Check sheet for the drawn part. Datum: minimum x, y, z corner. Units: mm. A direction names the side the tool comes from. Round coordinates to 2 decimals unless told otherwise and drop trailing zeros. Order: outer loops, then holes, each group sorted by start corner. A loop starts at its lowest first (then second) coordinate and runs counter-clockwise, first axis right, second up. Notation, with made-up numbers: (74.5, -36) -> (122.5, -36) arc R20 ccw to (122.5, -26) -> close; hole circle Ø3 at (81, 21). An arc over 180 degrees is marked (long way). Answer in a Markdown table with one row per item.
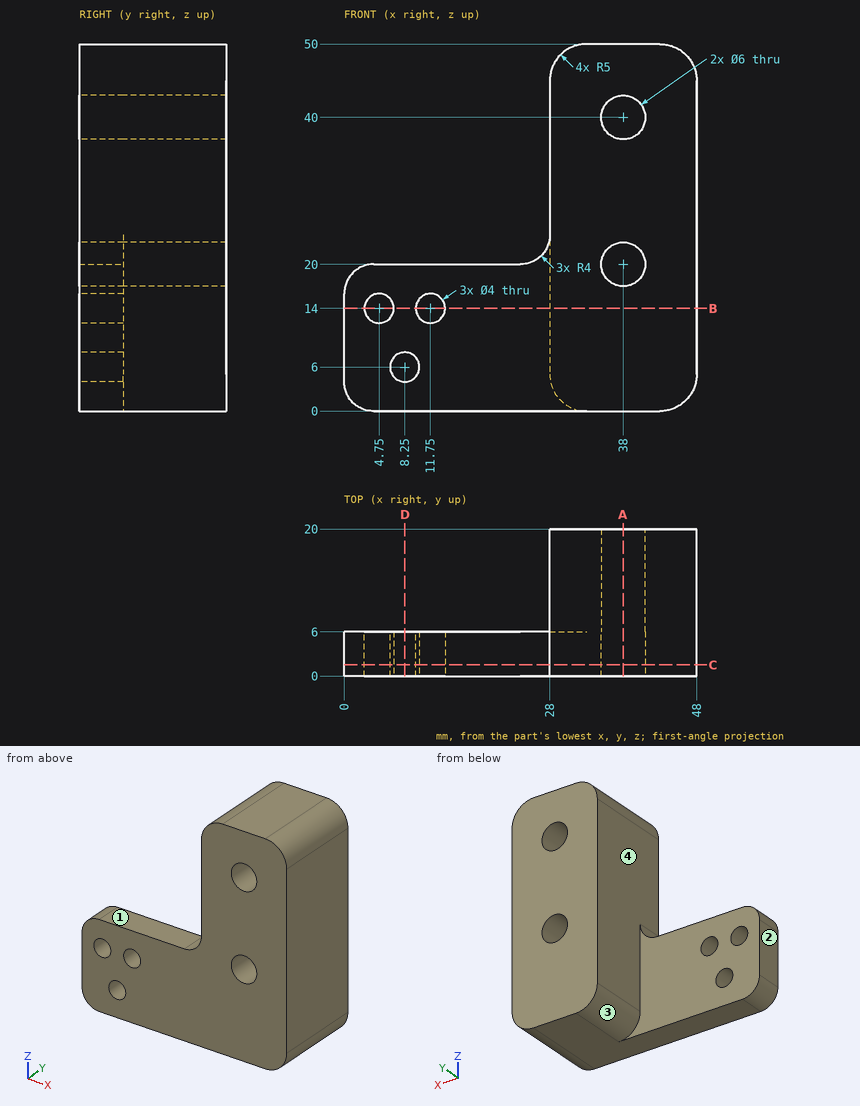
(1) Tool access check on the marked faces 1, 2, 3 and 4. Record the directions out of +Z, -Z, +X, -X, +Y, -Y that give a thin tool (end or side, any length) a straight path to the whole face; none if there is none.
Solutions:
| item | result |
|---|---|
| face 1 | +Z, -X, +Y, -Y |
| face 2 | +Z, -Z, -X, +Y, -Y |
| face 3 | -Z, -X, +Y |
| face 4 | +Z, -X, +Y |
(2) Section check C-C on y = 1.5. Record the boundary of the cut face in (x, z), plus the area to 3 significant figures.
Solutions:
| item | result |
|---|---|
| outline | (0, 4) arc R4 ccw to (4, 0) -> (43, 0) arc R5 ccw to (48, 5) -> (48, 45) arc R5 ccw to (43, 50) -> (33, 50) arc R5 ccw to (28, 45) -> (28, 24) arc R4 cw to (24, 20) -> (4, 20) arc R4 ccw to (0, 16) -> close; hole circle Ø4 at (4.75, 14); hole circle Ø4 at (8.25, 6); hole circle Ø4 at (11.75, 14); hole circle Ø6 at (38, 20); hole circle Ø6 at (38, 40) |
| area | 1,450 mm^2 |
(3) Section check D-D on x = 8.25. Record the boundary of the cut face in (y, z), plus the area to 3 significant figures.
Solutions:
| item | result |
|---|---|
| outline | (0, 0) -> (6, 0) -> (6, 4) -> (0, 4) -> close; (0, 8) -> (6, 8) -> (6, 20) -> (0, 20) -> close |
| area | 96.0 mm^2 |
(4) Section check B-B on z = 14. Record the boundary of the cut face in (x, y).
Solutions:
| item | result |
|---|---|
| outline | (0, 0) -> (2.75, 0) -> (2.75, 6) -> (0, 6) -> close; (6.75, 0) -> (9.75, 0) -> (9.75, 6) -> (6.75, 6) -> close; (13.75, 0) -> (48, 0) -> (48, 20) -> (28, 20) -> (28, 6) -> (13.75, 6) -> close |
(5) Scan lines: probe 1 along Z at (x, y) = (38, 3.5); probe 2 along X at (y, z) = (9.5, 40); probe 3 along X at (y, z) = (1.5, 6). Record each from-to range of solid material in increasing order. Write a range as from..to.
Solutions:
| item | result |
|---|---|
| probe 1 | 0..17, 23..37, 43..50 |
| probe 2 | 28..35, 41..48 |
| probe 3 | 0..6.25, 10.25..48 |
(6) Section check A-A on x = 38. Record the boundary of the cut face in (y, z).
Solutions:
| item | result |
|---|---|
| outline | (0, 0) -> (20, 0) -> (20, 17) -> (0, 17) -> close; (0, 23) -> (20, 23) -> (20, 37) -> (0, 37) -> close; (0, 43) -> (20, 43) -> (20, 50) -> (0, 50) -> close |
(7) Depth check by flat-ended pin: pin 1 Ø6 at (x, y) = (14.5, 5.5) entering from -Z; pin 2 Ø6 at (y, z) = (14, 38) entering from -X; pin 3 Ø10 at (x, z) = (16, 28.5) entering from +Y; pin 4 Ø1.5 at (x, z) = (21, 7.5) entering from +Y. Enter the tip coordinate at first touch or a pass-through.
Solutions:
| item | result |
|---|---|
| pin 1 | z = 0 |
| pin 2 | x = 28 |
| pin 3 | through |
| pin 4 | y = 6 |
